The drawing under review shows one solid part. Ordinate dimensions are in mm from its lowest x, y, z. Coordinates: 2 decimals unless noted, no trailing zeros. Order: outer loops, then holes, each group sorted by start corner. A loop starts at its lowest first (then second) coordinate and runs counter-clockwise, first axis right, second up. Notation, with made-up numbers: (57, -10) -> (80, -10) arc R32 cw to (80, 17) -> close; hole circle Ø1 at (62.5, 77). An arc over 180 degrees is marked (long way). Put each result on its own line as item: value.
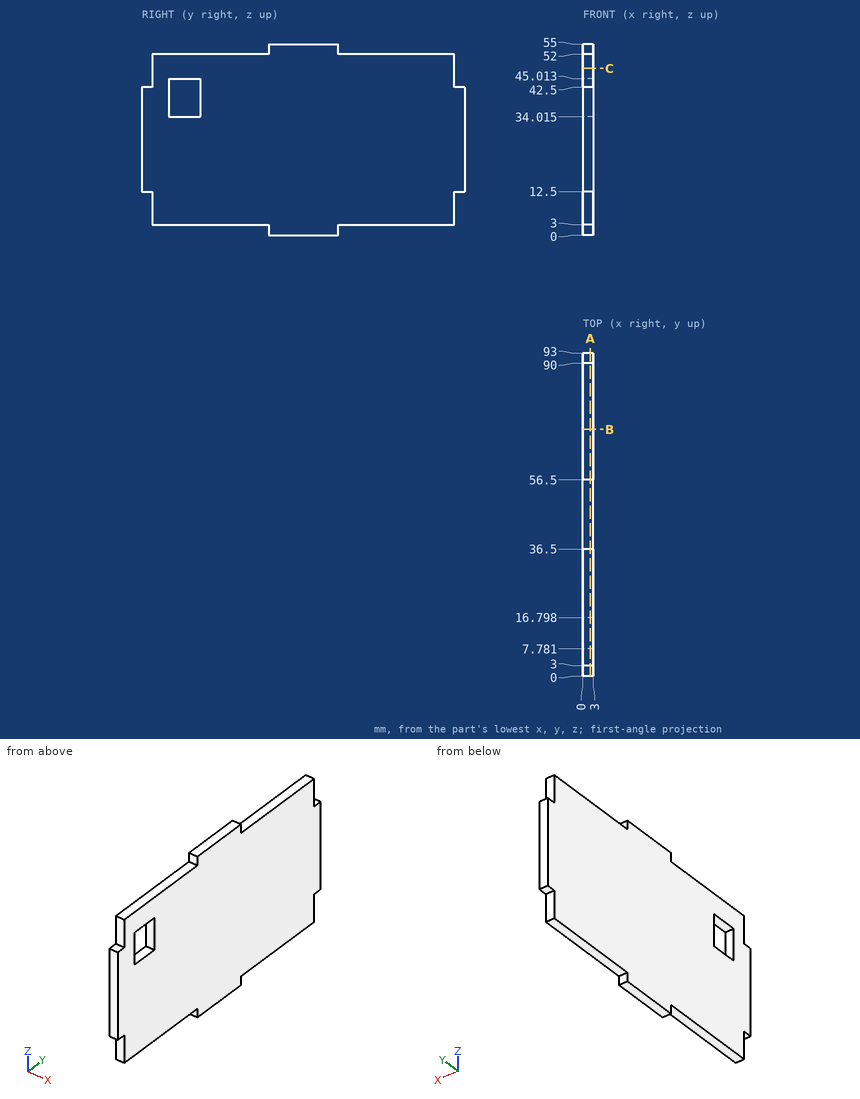
Item 1: Consider section C-C on z = 48. Write out the cut boundary in (x, y).
Answers below:
outline: (0, 3) -> (3, 3) -> (3, 90) -> (0, 90) -> close
Item 2: For pin 1 Ø6 at (y, z) = (51, 28.5) entering from -X; pin 2 Ø0.9 at (x, y) = (2, 14) entering from +Z; pin 3 Ø1.5 at (x, z) = (1, 49.5) entering from -Y; pin 4 Ø1.5 at (x, z) = (1.5, 2) entering from -Y, all flat-tipped, find the tip position at first contact; note any pin that passes through.
Answers below:
pin 1: x = 0
pin 2: z = 52
pin 3: y = 3
pin 4: y = 36.5
Item 3: Consider section B-B on y = 71. Write out the cut boundary in (x, z), and give its area (3 significant figures).
Answers below:
outline: (0, 3) -> (3, 3) -> (3, 52) -> (0, 52) -> close
area: 147 mm^2
Item 4: For line 1 (Y direction, x = 1.1, z = 34.5); line 2 (Z direction, x = 0.35, y = 82); line 3 (Y direction, x = 1.95, z = 47), list the stretches that pass through material, from the lowest coordinate up. Write a range as from..to.
Answers below:
line 1: 0..7.78, 16.8..93
line 2: 3..52
line 3: 3..90
Item 5: Consider section A-A on x = 2.15. Write out the cut boundary in (y, z) (1 decimal).
Answers below:
outline: (0, 12.5) -> (3, 12.5) -> (3, 3) -> (36.5, 3) -> (36.5, 0) -> (56.5, 0) -> (56.5, 3) -> (90, 3) -> (90, 12.5) -> (93, 12.5) -> (93, 42.5) -> (90, 42.5) -> (90, 52) -> (56.5, 52) -> (56.5, 55) -> (36.5, 55) -> (36.5, 52) -> (3, 52) -> (3, 42.5) -> (0, 42.5) -> close; hole (7.8, 34) -> (16.8, 34) -> (16.8, 45) -> (7.8, 45) -> close
